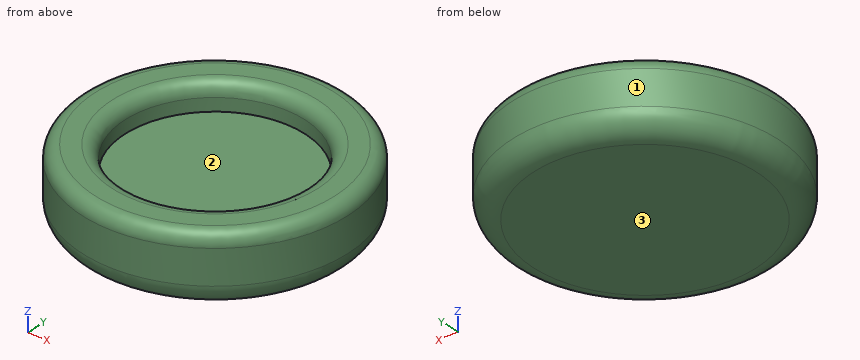
from build123d import *

# Parameters (mm, degrees)
F0_R     = 15.5
F1_DEPTH = 8
F2_T     = -5
F3_R     = 1.5
F4_R     = 2.5


with BuildPart() as f1:
    # F0 (on Top) → F1 (new body)
    with BuildSketch(Plane.XY):
        with Locations((-13.3484182879, 0)):
            Circle(F0_R)
    extrude(amount=F1_DEPTH)

    # F2
    f2_openings = [f1.faces().sort_by_distance(p)[0] for p in [
        (-13.348418, 0, 8),
    ]]
    offset(amount=F2_T, openings=f2_openings)

    # F3
    f3_edges = [f1.edges().sort_by_distance(p)[0] for p in [
        (-28.848418, 0, 8),
        (-23.848418, 0, 8),
    ]]
    fillet(f3_edges, radius=F3_R)

    # F4
    f4_edges = [f1.edges().sort_by_distance(p)[0] for p in [
        (-28.848418, 0, 0),
    ]]
    fillet(f4_edges, radius=F4_R)


solid = f1.part
Model file for the job. Use its own axes, mm. Face numbers are marked on the shaded views. Give positions to 0.01 mm unless a question says otherwise; leave off trailing zeros. Loops run counter-clockwise (first coordinate to the right, second up) from the corner with the lowest first, then second, coordinate; pieces in that order, holes last. Notation, with made-up numbers: (24, 16.5) -> (55, 16.5) arc R17 cw to (55, 49.5) -> close; hole circle Ø3 at (-34, 18.25). An arc over 180 degrees is marked (long way). Use a Markdown table: item, result. Add a question column.
(1) Slice it at D-D on z = 1.75. List the corners of the cut face in (x, y).
(2) Mould opens along Y. For the marked faces 1, 2 and 3 say: +Y half, -Y half, draft (parallel to the pull), parting line (faces both ways), or undercut.
(3) Wall check: line 1 along Y through (x, z) = (-13, 6); line 2 along Z through (x, y) = (-20, -6.5); line 3 along X through (y, z) = (-7.5, 6.5). Give the ranges that are in metal, low to high.
(4) Slice it at C-C on z = 7. List the corners of the cut face in (x, y).
(5) Drop flat-ended pins along their axis: pin 1 Ø3 at (y, z) = (11.5, 3.5) entering from +X; pin 2 Ø2 at (y, z) = (7.5, 5.5) entering from +X; pin 3 Ø2 at (x, z) = (-24.5, 2.5) entering from -Y; pin 4 Ø3 at (x, y) = (-15.5, -0.5) entering from -Z. Give the stop position or say it passes through.
(6) Slice it at A-A on y = 0. List the corners of the cut face in (x, z), and give its area (3 significant figures).
(7) Slice it at B-B on z = 3.5. List the corners of the cut face in (x, y), and give its area (3 significant figures).
Filled sheet:
| question | item | result |
|---|---|---|
| 1 | outline | circle Ø30.77 at (-13.35, 0) |
| 2 | face 1 | parting line |
| 2 | face 2 | undercut |
| 2 | face 3 | draft |
| 3 | line 1 | -15.5 to -10.49, 10.49 to 15.5 |
| 3 | line 2 | 0 to 5 |
| 3 | line 3 | -26.91 to -20.7, -6 to 0.22 |
| 4 | outline | circle Ø30.83 at (-13.35, 0); hole circle Ø21.17 at (-13.35, 0) |
| 5 | pin 1 | x = -1.51 |
| 5 | pin 2 | x = 0.72 |
| 5 | pin 3 | y = -11.71 |
| 5 | pin 4 | z = 0 |
| 6 | outline | (-28.85, 2.5) arc R2.5 ccw to (-26.35, 0) -> (-0.35, 0) arc R2.5 ccw to (2.15, 2.5) -> (2.15, 6.5) arc R1.5 ccw to (0.65, 8) -> (-1.35, 8) arc R1.5 ccw to (-2.85, 6.5) -> (-2.85, 5) -> (-23.85, 5) -> (-23.85, 6.5) arc R1.5 ccw to (-25.35, 8) -> (-27.35, 8) arc R1.5 ccw to (-28.85, 6.5) -> close |
| 6 | area | 180 mm2 |
| 7 | outline | circle Ø31 at (-13.35, 0) |
| 7 | area | 755 mm2 |
